Design review of the part built by this model. Coordinates are the model's own, in mm. Face numbers are marked on the shaded views. A direction names the side the tool comes from. Coordinates: 2 decimals unless noted, no trailing zeros. Loops run counter-clockwise (first coordinate to the right, second up) from the corner with the lowest first, then second, coordinate; pieces in that order, holes last. Notation, with made-up numbers: M 67.5,-22 L 76.5,-22 A15 cw 76.5,-9 Z; hole C -3.75,17.5 d7. An arc over 180 degrees is marked long. Answer as a JSON object with one key per item and string values. Group by question number.
1. Consider section A-A (y = 0). State the section outline as (x, z) points (3 decimals).
2. Insertion check: pin 1 (1.8 mm diameter, centred on x = -11.557, y = -11.557, fed in from +Z); pin 2 (0.6 mm diameter, centred on x = -0.5, z = 2, fed in from -Y) (3 decimals); pin 3 (3 mm diameter, centred on x = -2, y = -3.5, fed in from +Z). Each pin has a flat end and moves straight along its axis. Give the tip position at first contact, or say it passes through.
3. Consider section B-B (x = 11.43). State the section outline as (y, z) points.
4. Consider section C-C (x = 0). State the section outline as (y, z) points (3 decimals), then the cut area to 3 significant figures.
5. Machinability: for the marked faces 1 and 2, which of the approach directions +Z, -Z, +X, -X, +Y, -Y give a long, thin tool a straight path to every point of the face, cutting with its end or side? Answer none if there is none.
6. To check wall thickness, follow probe 1 along X at (y, z) = (11, 0.6); probe 2 along X at (y, z) = (11.5, 1.1); probe 3 along Z at (x, y) = (7, -9.5). State the ranges of each line that lie inside material, in increasing order.
7. Consider section D-D (y = -4.5). State the section outline as (x, z) points.
from build123d import *

# Parameters (mm, degrees)
SKETCH1_R           = 17.78
BOSS_EXTRUDE1_DEPTH = 1.6256
SKETCH2_R           = 0.508
CUT_EXTRUDE1_DEPTH  = 26.197209674
SKETCH3_W           = 6.35
SKETCH3_H           = 6.35
BOSS_EXTRUDE2_DEPTH = 0.762
SKETCH4_R           = 1.143
BOSS_EXTRUDE3_DEPTH = 0.762
SKETCH5_R           = 0.7874
CUT_EXTRUDE2_DEPTH  = 26.197209674


with BuildPart() as part:
    # Sketch1 → Boss-Extrude1 (new body)
    with BuildSketch(Plane.XY):
        Circle(SKETCH1_R)
    extrude(amount=BOSS_EXTRUDE1_DEPTH)

    # Sketch2 → Cut-Extrude1 (cut, through all)
    with BuildSketch(Plane.XY.offset(1.6256)):
        with Locations((-11.43, 0)):
            Circle(SKETCH2_R)
        with Locations((11.43, 0)):
            Circle(SKETCH2_R)
    extrude(amount=-CUT_EXTRUDE1_DEPTH, mode=Mode.SUBTRACT)

    # Sketch3 → Boss-Extrude2 (add)
    with BuildSketch(Plane.XY.offset(1.6256)):
        Rectangle(SKETCH3_W, SKETCH3_H)
    extrude(amount=BOSS_EXTRUDE2_DEPTH)

    # Sketch4 → Boss-Extrude3 (add)
    with BuildSketch(Plane.XY.offset(2.3876)):
        with Locations(Location((0, 0, 0), (0, 0, 180))):
            Circle(SKETCH4_R)
    extrude(amount=BOSS_EXTRUDE3_DEPTH)

    # Sketch5 → Cut-Extrude2 (cut, through all)
    with BuildSketch(Plane.XY.offset(1.6256)):
        with Locations((-11.557, 11.557)):
            Circle(SKETCH5_R)
        with Locations((11.557, 11.557)):
            Circle(SKETCH5_R)
        with Locations((11.557, -11.557)):
            Circle(SKETCH5_R)
        with Locations((-11.557, -11.557)):
            Circle(SKETCH5_R)
    extrude(amount=-CUT_EXTRUDE2_DEPTH, mode=Mode.SUBTRACT)


solid = part.part
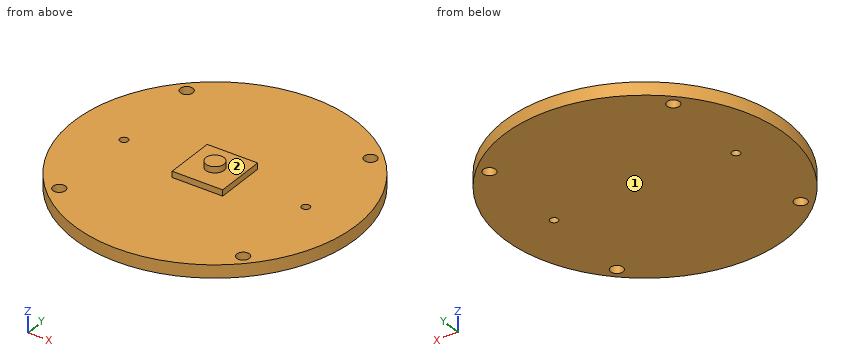
Findings below:
{
 "1": {"outline": "M -17.78,0 L -11.938,0 L -11.938,1.626 L -17.78,1.626 Z; M -10.922,0 L 10.922,0 L 10.922,1.626 L 3.175,1.626 L 3.175,2.388 L 1.143,2.388 L 1.143,3.15 L -1.143,3.15 L -1.143,2.388 L -3.175,2.388 L -3.175,1.626 L -10.922,1.626 Z; M 11.938,0 L 17.78,0 L 17.78,1.626 L 11.938,1.626 Z"},
 "2": {"pin 1": "stops at z = 1.63", "pin 2": "stops at y = -3.175", "pin 3": "stops at z = 2.39"},
 "3": {"outline": "M -13.62,0 L -12.33,0 L -12.33,1.63 L -13.62,1.63 Z; M -10.78,0 L -0.51,0 L -0.51,1.63 L -10.78,1.63 Z; M 0.51,0 L 10.78,0 L 10.78,1.63 L 0.51,1.63 Z; M 12.33,0 L 13.62,0 L 13.62,1.63 L 12.33,1.63 Z"},
 "4": {"outline": "M -17.78,0 L 17.78,0 L 17.78,1.626 L 3.175,1.626 L 3.175,2.388 L 1.143,2.388 L 1.143,3.15 L -1.143,3.15 L -1.143,2.388 L -3.175,2.388 L -3.175,1.626 L -17.78,1.626 Z", "area": "64.4 mm^2"},
 "5": {"face 1": "-Z, +X, -X, +Y, -Y", "face 2": "+Z"},
 "6": {"probe 1": "x = -13.97 to -12.11, -11 to 11, 12.11 to 13.97", "probe 2": "x = -13.56 to -12.34, -10.77 to 10.77, 12.34 to 13.56", "probe 3": "z = 0 to 1.63"},
 "7": {"outline": "M -17.2,0 L 17.2,0 L 17.2,1.63 L -17.2,1.63 Z"}
}
